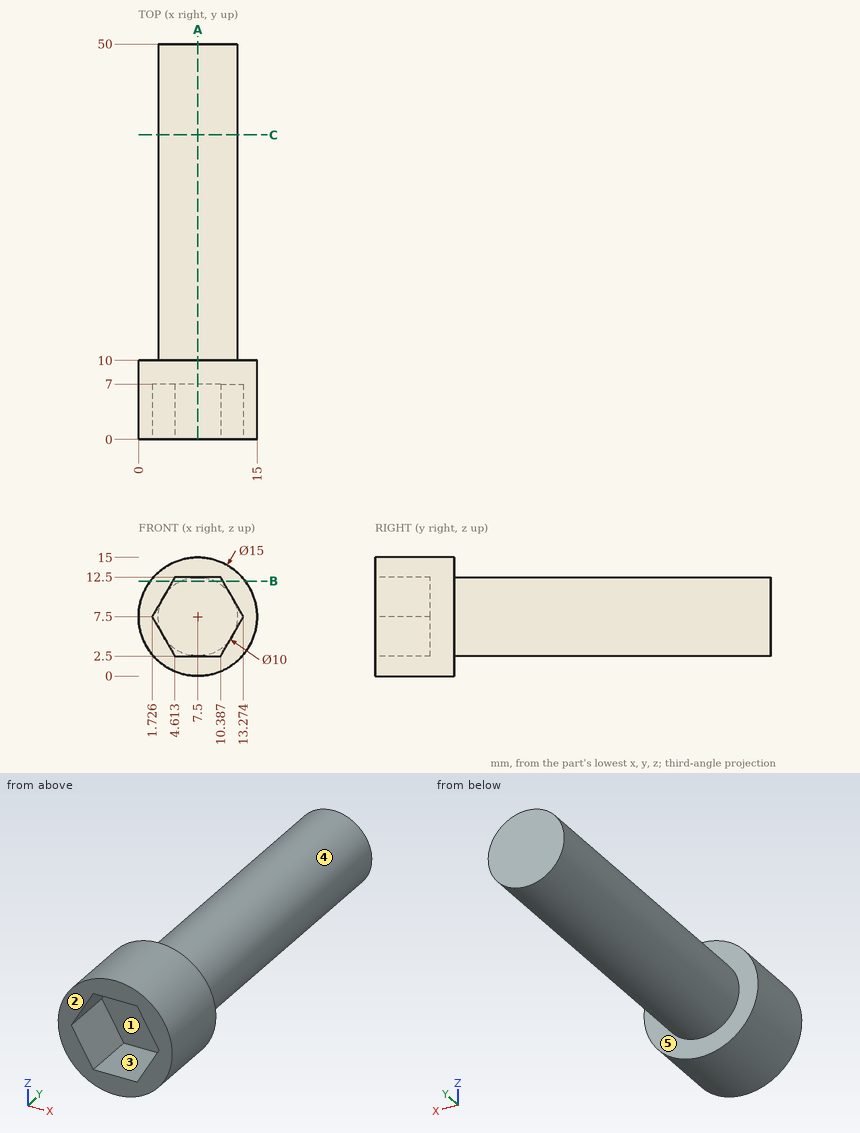
Check sheet for the drawn part. Datum: minimum x, y, z corner. Units: mm. A direction names the side the tool comes from. Give positions to 0.01 mm unless a question says otherwise; leave off trailing zeros. Write each loop counter-clockwise with the first axis right and the second up, starting at its lowest first coordinate (ties: lowest second). Pieces come first, ordered by that corner, then holes.
(1) Mould release check, pull along Z, two halves, no side actions. Record for the marked faces 3, 4 and 5: +Z half, -Z half, draft (parallel to the pull), parting line (faces both ways), or undercut.
(2) Cross-section at C-C (y = 38.5). Enter the section's corners in (x, z).
(3) Gauge pin test, flat ends, axial feed: pin 1 (6 mm diameter, centred on x = 9, y = 31.5, fed in from -Z); pin 2 (1 mm diameter, centred on y = 8.5, z = 8.5, fed in from +X); pin 3 (6 mm diameter, centred on y = 42.5, z = 11.5, fed in from -X); pin 4 (6.5 mm diameter, centred on x = 7, y = 4.5, fed in from -Z). Record the tip position at first contact, or that the pin passes through.
(4) Cross-section at B-B (z = 12). Enter the section's corners in (x, y) (1 decimal).
(5) Access from +Z, -Z, +X, -X, +Y, -Y to the whole of each face (thin tool, end or side, straight path). Record for the marked faces 1 and 2.
(6) Material ranges on line 1 (Y direction, x = 11, z = 10); line 2 (Y direction, x = 1.5, z = 11); line 3 (Z direction, x = 8, y = 44) (1 decimal), recorded low to high.
(7) Cross-section at A-A (x = 7.5). Enter the section's corners in (y, z).
Worked out:
1. face 3: undercut
1. face 4: parting line
1. face 5: draft
2. outline: circle Ø10 at (7.5, 7.5)
3. pin 1: stops at z = 2.5
3. pin 2: stops at x = 14.98
3. pin 3: stops at x = 2.6
3. pin 4: stops at z = 0
4. outline: (1.5, 0) - (4.3, 0) - (4.3, 7) - (10.7, 7) - (10.7, 0) - (13.5, 0) - (13.5, 10) - (9.7, 10) - (9.7, 50) - (5.3, 50) - (5.3, 10) - (1.5, 10) - close
5. face 1: -Y
5. face 2: +Z, -Z, +X, -X, -Y
6. line 1: y = 7 to 50
6. line 2: y = 0 to 10
6. line 3: z = 2.5 to 12.5
7. outline: (0, 0) - (10, 0) - (10, 2.5) - (50, 2.5) - (50, 12.5) - (10, 12.5) - (10, 15) - (0, 15) - (0, 12.5) - (7, 12.5) - (7, 2.5) - (0, 2.5) - close
